CAD build for the part. Positions are in the model's coordinates, mm. A direction names the side the tool comes from. Give positions to 0.01 mm unless a question says otherwise; leave off trailing zeros. Write each loop counter-clockwise with the first axis right and the second up, starting at its lowest first coordinate (ties: lowest second). Pieces come first, ordered by that corner, then holes. Notation, with made-up numbers: (67, 77) - (79, 77) arc R14 cw to (79, 100) - close; hole circle Ø1 at (64, -26.75). An arc over 180 degrees is marked (long way). Answer as a JSON object with one key per item and string values.
Autodesk Fusion 360 part; units mm, degrees
sketch "Sketch1" plane through (0, 0, 0) normal (0, 0, 1) x (1, 0, 0)
  line L0 (0, 0) -> (0, 28) construction
  line L1 (0, 28) -> (21, 28) construction
  line L2 (21, 28) -> (0, 28) construction
  line L3 (0, 28) -> (0, 0) construction
  line L4 (0, 0) -> (21, 0) construction
  line L5 (21, 0) -> (21, 28) construction
  line L6 (10.5, 0) -> (10.5, 28) construction
  line L7 (10.5, 0) -> (10.5, 2) construction
  line L8 (10.5, 28) -> (10.5, 26) construction
  circle A0 centre (10.5, 26) radius 1.25 construction
  circle A1 centre (10.5, 2) radius 1.25 construction
  line L9 (21, 28) -> (0, 28)
  line L10 (0, 28) -> (0, 0)
  line L11 (0, 0) -> (21, 0)
  line L12 (21, 0) -> (21, 28)
  circle A2 centre (10.5, 2) radius 1.25
  circle A3 centre (10.5, 26) radius 1.25
  dimension "d38" = 28
  dimension "d39" = 21
  dimension "d40" = 2
  dimension "d41" = 2
  dimension "d42" = 2.5
  dimension "d43" = 2.5
extrude "Extrude1" add sketch "Sketch1" along normal blind 1.6
sketch "Sketch2" plane through (0, 0, 1.6) normal (0, 0, 1) x (-1, 0, 0)
  circle A0 centre (-10.5, -26) radius 1.25
  circle A1 centre (-10.5, -2) radius 1.25
  line L0 (-21, 0) -> (-21, -28)
  line L1 (-21, -28) -> (0, -28)
  line L2 (0, -28) -> (0, 0)
  line L3 (0, 0) -> (-21, 0)
  line L4 (0, -14) -> (-21, -14) construction
  line L5 (-10.5, -28) -> (-10.5, 0) construction
  line L6 (-10.5, -14) -> (-10.5, -24.5) construction
  line L7 (-10.5, -24.5) -> (-19.85, -24.5) construction
  line L8 (-10.5, -14) -> (-10.5, -3.5) construction
  line L9 (-10.5, -3.5) -> (-1.15, -3.5) construction
  line L10 (-1.15, -3.5) -> (-19.85, -3.5) construction
  line L11 (-19.85, -3.5) -> (-19.85, -24.5) construction
  line L12 (-19.85, -24.5) -> (-1.15, -24.5) construction
  line L13 (-1.15, -24.5) -> (-1.15, -3.5) construction
  line L14 (-1.15, -3.5) -> (-19.85, -3.5)
  line L15 (-19.85, -3.5) -> (-19.85, -24.5)
  line L16 (-19.85, -24.5) -> (-1.15, -24.5)
  line L17 (-1.15, -24.5) -> (-1.15, -3.5)
  dimension "d46" = 10.5
  dimension "d47" = 9.35
  dimension "d48" = 10.5
  dimension "d49" = 9.35
extrude "Extrude2" add sketch "Sketch2" along normal blind 3.5 contours L14 L15 L16 L17
fillet "Fillet1" radius 6 4 edges at (19.85, 3.5, 3.35) (1.15, 3.5, 3.35) (1.15, 24.5, 3.35) (19.85, 24.5, 3.35)
(1) Saw through at D-D, the plane y = 11.5. Give the cut face in (x, z).
Answer key:
{"outline": "(0, 0) - (21, 0) - (21, 1.6) - (19.85, 1.6) - (19.85, 5.1) - (1.15, 5.1) - (1.15, 1.6) - (0, 1.6) - close"}
(2) Probe L1, parallel to Y at x = 10.5, z = 1.05; L2, parallel to Z at x = 18.5, y = 3; L3, parallel to Y at x = 13.75, z = 4. List the from-to ranges inside material, lowest first. Write a range as [from, to].
Answer key:
{"L1": "y = [0, 0.75], [3.25, 24.75], [27.25, 28]", "L2": "z = [0, 1.6]", "L3": "y = [3.5, 24.5]"}
(3) Flat gauge pins, fed straight in: P1, Ø3, axis at y = 12, z = 3.5, coming from the +X side; P2, Ø1.7, axis at x = 11, z = 3.5, coming from the +Y side. Where does each tip first touch, or does it go through?
Answer key:
{"P1": "stops at x = 19.85", "P2": "stops at y = 24.5"}
(4) 3-axis set-ups, long thin cutter, end or side, ignore diameter. For faces 1 (the face through (2.954, 22.789, 3.374)), 2 (the face through (10, 3.5, 3)), 3 (the face through (0.3, 15.1, 1.6)), 4 (the face through (18.046, 5.211, 3.374)), 5 (the face through (2.861, 5.304, 3.374)): which of +Z, -Z, +X, -X, +Y, -Y reach the whole face in a straight line?
Answer key:
{"face 1": "+Z, -X, +Y", "face 2": "+Z, +X, -X, -Y", "face 3": "+Z", "face 4": "+Z, +X, -Y", "face 5": "+Z, -X, -Y"}
(5) Saw through at C-C, the plane z = 1.95. Give the cut face in (x, y).
Answer key:
{"outline": "(1.15, 9.5) arc R6 ccw to (7.15, 3.5) - (13.85, 3.5) arc R6 ccw to (19.85, 9.5) - (19.85, 18.5) arc R6 ccw to (13.85, 24.5) - (7.15, 24.5) arc R6 ccw to (1.15, 18.5) - close"}
(6) Saw through at A-A, the plane x = 10.5. Give the cut face in (y, z).
Answer key:
{"outline": "(0, 0) - (0.75, 0) - (0.75, 1.6) - (0, 1.6) - close; (3.25, 0) - (24.75, 0) - (24.75, 1.6) - (24.5, 1.6) - (24.5, 5.1) - (3.5, 5.1) - (3.5, 1.6) - (3.25, 1.6) - close; (27.25, 0) - (28, 0) - (28, 1.6) - (27.25, 1.6) - close"}
(7) Pull direction Y, two halves, no side cores. Call faces 6 (the face through (9.51, 26.76, 0.79)), 7 (the face through (11, 14, 5.1)), 8 (the face through (10, 0, 1)): pulls with the +Y half, pulls with the -Y half, needs draft (parallel to the pull), parting line crosses it, or undercut.
Answer key:
{"face 6": "undercut", "face 7": "needs draft", "face 8": "pulls with the -Y half"}
(8) Saw through at B-B, the plane y = 2. Give the cut face in (x, z).
Answer key:
{"outline": "(0, 0) - (9.25, 0) - (9.25, 1.6) - (0, 1.6) - close; (11.75, 0) - (21, 0) - (21, 1.6) - (11.75, 1.6) - close"}
